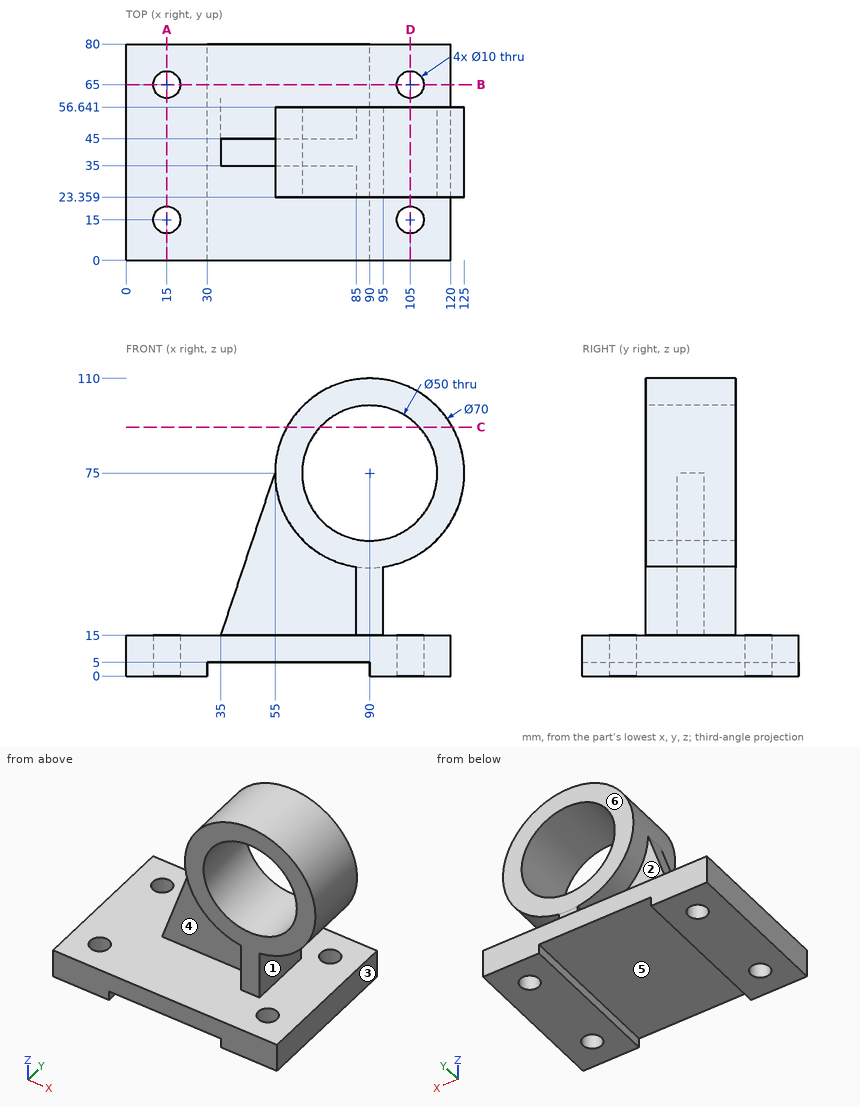
Input: dimensioned drawing with shaded views. Units: mm. Origin: part minimum x, y, z. A direction names the side the tool comes from. Coordinates: 2 decimals unless noted, no trailing zeros. Loops run counter-clockwise (first coordinate to the right, second up) from the corner with the lowest first, then second, coordinate; pieces in that order, holes last. Notation, with made-up numbers: (71.5, 25.25) - (80.5, 25.25) arc R19 ccw to (80.5, 44.25) - close; hole circle Ø2 at (-29.75, 59). An arc over 180 degrees is marked (long way). One line per question, with ' | ' between items. Start each with the question number.
(1) Cut plane A-A on x = 15. Output: boundary loops of the cut face in (y, z).
(2) Draft query along Z for the marked faces 4, 5 and 6. Return one class per face: +Z half, -Z half, draft (parallel to the pull), parting line (faces both ways), or undercut.
(3) First-contact query: pin 1 (16 mm diameter, centred on x = 15, y = 15, fed in from +Z); pin 2 (5 mm diameter, centred on x = 88.5, z = 28, fed in from +Y); pin 3 (15 mm diameter, centred on x = 64, z = 35.5, fed in from +Y); pin 4 (4 mm diameter, centred on y = 59, z = 55, fed in from +X). Flat tips, straight axial feed; report the tip coordinate or a pass-through.
(4) Cut plane B-B on y = 65. Output: boundary loops of the cut face in (x, z), and give its area (3 significant figures).
(5) Ray query, L1, parallel to Y at x = 105, z = 10; L2, parallel to Z at x = 106.5, y = 56.5; L3, parallel to Y at x = 53.5, z = 49. Return the intervals inside material, ascending. Write a range as from..to.
(6) Cut plane C-C on z = 92. Output: boundary loops of the cut face in (x, y), and give its area (3 significant figures).
(7) Reachability of the marked faces 1, 2 and 3 from +Z, -Z, +X, -X, +Y, -Y: full face, straight path, thin tool, end or side. Return the list, or none.
(8) Cut plane D-D on x = 105. Output: boundary loops of the cut face in (y, z).
Here are the results:
1) outline: (0, 0) - (10, 0) - (10, 15) - (0, 15) - close; (20, 0) - (60, 0) - (60, 15) - (20, 15) - close; (70, 0) - (80, 0) - (80, 15) - (70, 15) - close
2) face 4: undercut | face 5: -Z half | face 6: draft
3) pin 1: z = 15 | pin 2: y = 56.64 | pin 3: y = 45 | pin 4: through
4) outline: (0, 0) - (10, 0) - (10, 15) - (0, 15) - close; (20, 0) - (30, 0) - (30, 5) - (90, 5) - (90, 0) - (100, 0) - (100, 15) - (20, 15) - close; (110, 0) - (120, 0) - (120, 15) - (110, 15) - close | area: 1,200 mm²
5) L1: 0..10, 20..60, 70..80 | L2: 0..15, 44.13..56.22, 93.78..105.87 | L3: 35..45
6) outline: (59.41, 23.36) - (71.67, 23.36) - (71.67, 56.64) - (59.41, 56.64) - close; (108.33, 23.36) - (120.59, 23.36) - (120.59, 56.64) - (108.33, 56.64) - close | area: 816 mm²
7) face 1: +X, +Y, -Y | face 2: -X, +Y | face 3: -Z, +X, +Y, -Y
8) outline: (0, 0) - (10, 0) - (10, 15) - (0, 15) - close; (20, 0) - (60, 0) - (60, 15) - (20, 15) - close; (23.36, 43.38) - (56.64, 43.38) - (56.64, 55) - (23.36, 55) - close; (23.36, 95) - (56.64, 95) - (56.64, 106.62) - (23.36, 106.62) - close; (70, 0) - (80, 0) - (80, 15) - (70, 15) - close
